Study the drawing (mm; zero at the part's minimum x, y, z) and answer. A direction names the side the tool comes from. Give positions to 0.01 mm unless a question says otherwise; leave off trailing zeros. Loops run counter-clockwise (first coordinate to the right, second up) from the corner with the lowest first, then second, coordinate; pieces in that order, holes last. Notation, with made-up numbers: M -1,-23.75 L 16,-23.75 A12 ccw 16,-17.75 Z; hole C 40,63.25 d5. An arc over 180 degrees is marked long. Return JSON: item names as keys, results as strings.
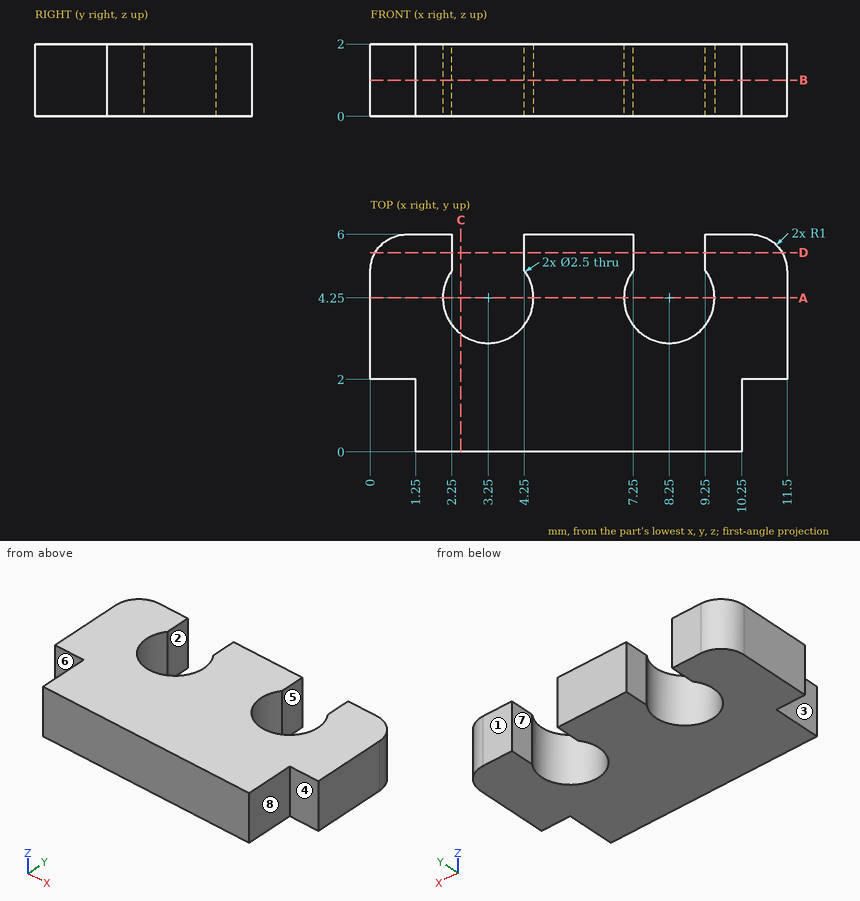
(1) Straight lines are drawn through the part: line 1 along X through (y, z) = (3.5, 1.75); line 2 along X through (y, z) = (4.25, 1); line 3 along Y through (x, z) = (8.25, 0.9). For each, find the intervals that lie inside material, in ascending order.
Values follow:
{"line 1": "0 to 2.25, 4.25 to 7.25, 9.25 to 11.5", "line 2": "0 to 2, 4.5 to 7, 9.5 to 11.5", "line 3": "0 to 3"}
(2) The part is cut by section D-D (y = 5.5). Determine the outline of the cut face in (x, z).
Values follow:
{"outline": "M 0.13,0 L 2.25,0 L 2.25,2 L 0.13,2 Z; M 4.25,0 L 7.25,0 L 7.25,2 L 4.25,2 Z; M 9.25,0 L 11.37,0 L 11.37,2 L 9.25,2 Z"}
(3) Given pin 1 (0.5 mm diameter, centred on y = 5.5, z = 1.5, fed in from -X); pin 2 (1 mm diameter, centred on x = 11, z = 1, fed in from -Y); pin 3 (0.6 mm diameter, centred on y = 1.5, z = 1, fed in from +X), each flat-ended and moving along its own axis, determine where each tip first touches the part or whether it passes through.
Values follow:
{"pin 1": "x = 0.03", "pin 2": "y = 2", "pin 3": "x = 10.25"}
(4) The part is cut by section A-A (y = 4.25). Determine the outline of the cut face in (x, z), and give its area (3 significant figures).
Values follow:
{"outline": "M 0,0 L 2,0 L 2,2 L 0,2 Z; M 4.5,0 L 7,0 L 7,2 L 4.5,2 Z; M 9.5,0 L 11.5,0 L 11.5,2 L 9.5,2 Z", "area": "13.0 mm²"}
(5) The part is cut by section C-C (x = 2.5). Determine the outline of the cut face in (y, z), and give its area (3 significant figures).
Values follow:
{"outline": "M 0,0 L 3.25,0 L 3.25,2 L 0,2 Z", "area": "6.50 mm²"}
(6) A tool of negligible diameter and unlimited length cuts with its end or side. For the marked faces 1, 2, 3 and 4, from which of +Z, -Z, +X, -X, +Y, -Y can it reach the whole face along a straight path? Write none if from no direction.
Values follow:
{"face 1": "+Z, -Z, +X, -X, +Y", "face 2": "+Z, -Z, +Y", "face 3": "+Z, -Z, -X, -Y", "face 4": "+Z, -Z, +X, -Y"}
(7) The part is cut by section B-B (z = 1). Determine the outline of the cut face in (x, y), and give its area (3 significant figures).
Values follow:
{"outline": "M 0,2 L 1.25,2 L 1.25,0 L 10.25,0 L 10.25,2 L 11.5,2 L 11.5,5 A1 ccw 10.5,6 L 9.25,6 L 9.25,5 A1.25 cw long 7.25,5 L 7.25,6 L 4.25,6 L 4.25,5 A1.25 cw long 2.25,5 L 2.25,6 L 1,6 A1 ccw 0,5 Z", "area": "51.2 mm²"}
(8) Determine the mould class of the marked faces 5, 6, 7 and 8 for opening direction X: released by +X, released by -X, zero draft, split by the parting line, or undercut.
Values follow:
{"face 5": "undercut", "face 6": "zero draft", "face 7": "undercut", "face 8": "released by +X"}
